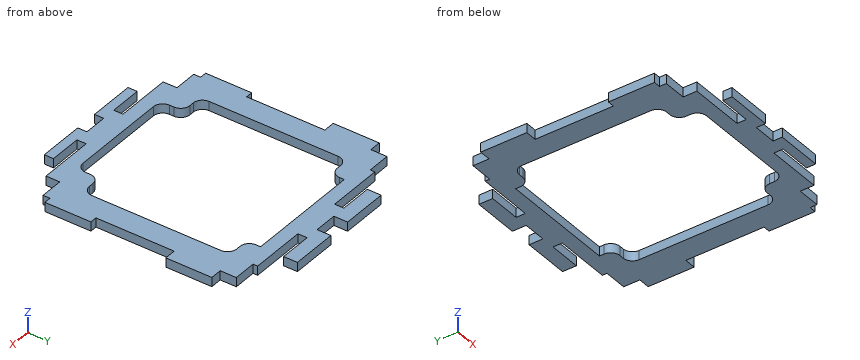
```python
from build123d import *

# Parameters (mm, degrees)
EXTRUDE_1_DEPTH = 2


with BuildPart() as part:
    # Model → 凸台-拉伸1 (new body)
    with BuildSketch(Plane.XY):
        Polygon((1277.912077, 487.080631391), (1277.912077, 483.580631391), (1275.412077, 483.580631391), (1275.412077, 473.580631391), (1277.912077, 473.580631391), (1277.912077, 456.580631391), (1276.412077, 456.580631391), (1276.412077, 446.580631391), (1277.912077, 446.580631391), (1277.912077, 445.080631391), (1282.912077, 445.080631391), (1282.912077, 442.080631391), (1294.912077, 442.080631391), (1294.912077, 440.080631391), (1287.912077, 440.080631391), (1287.912077, 438.080631391), (1297.912077, 438.080631391), (1297.912077, 440.080631391), (1302.912077, 440.080631391), (1302.912077, 438.080631391), (1312.912077, 438.080631391), (1312.912077, 440.080631391), (1305.912077, 440.080631391), (1305.912077, 442.080631391), (1317.912077, 442.080631391), (1317.912077, 445.080631391), (1322.912077, 445.080631391), (1322.912077, 446.580631391), (1324.412077, 446.580631391), (1324.412077, 456.580631391), (1322.912077, 456.580631391), (1322.912077, 473.580631391), (1325.412077, 473.580631391), (1325.412077, 483.580631391), (1322.912077, 483.580631391), (1322.912077, 487.080631391), (1317.912077, 487.080631391), (1317.912077, 488.080631391), (1305.912077, 488.080631391), (1305.912077, 490.080631391), (1312.912077, 490.080631391), (1312.912077, 493.080631391), (1302.912077, 493.080631391), (1302.912077, 490.080631391), (1297.912077, 490.080631391), (1297.912077, 493.080631391), (1287.912077, 493.080631391), (1287.912077, 490.080631391), (1294.912077, 490.080631391), (1294.912077, 488.080631391), (1282.912077, 488.080631391), (1282.912077, 487.080631391), align=None)
        with BuildLine():
            Line((1284.912077, 482.080631391), (1285.912077, 482.080631391))
            ThreePointArc((1285.912077, 482.080631391), (1287.326290562, 482.666417828), (1287.912077, 484.080631391))
            Line((1287.912077, 484.080631391), (1287.912077, 485.080631391))
            Line((1287.912077, 485.080631391), (1312.912077, 485.080631391))
            Line((1312.912077, 485.080631391), (1312.912077, 484.080631391))
            ThreePointArc((1312.912077, 484.080631391), (1313.497863438, 482.666417828), (1314.912077, 482.080631391))
            Line((1314.912077, 482.080631391), (1315.912077, 482.080631391))
            ThreePointArc((1315.912077, 482.080631391), (1317.326290562, 481.494844953), (1317.912077, 480.080631391))
            Line((1317.912077, 480.080631391), (1317.912077, 452.080631391))
            ThreePointArc((1317.912077, 452.080631391), (1317.326290562, 450.666417828), (1315.912077, 450.080631391))
            Line((1315.912077, 450.080631391), (1314.912077, 450.080631391))
            ThreePointArc((1314.912077, 450.080631391), (1313.497863438, 449.494844953), (1312.912077, 448.080631391))
            Line((1312.912077, 448.080631391), (1312.912077, 447.080631391))
            ThreePointArc((1312.912077, 447.080631391), (1312.326290562, 445.666417828), (1310.912077, 445.080631391))
            Line((1310.912077, 445.080631391), (1289.912077, 445.080631391))
            ThreePointArc((1289.912077, 445.080631391), (1288.497863438, 445.666417828), (1287.912077, 447.080631391))
            Line((1287.912077, 447.080631391), (1287.912077, 448.080631391))
            ThreePointArc((1287.912077, 448.080631391), (1287.326290562, 449.494844953), (1285.912077, 450.080631391))
            Line((1285.912077, 450.080631391), (1284.912077, 450.080631391))
            ThreePointArc((1284.912077, 450.080631391), (1283.497863438, 450.666417828), (1282.912077, 452.080631391))
            Line((1282.912077, 452.080631391), (1282.912077, 480.080631391))
            ThreePointArc((1282.912077, 480.080631391), (1283.497863438, 481.494844953), (1284.912077, 482.080631391))
        make_face(mode=Mode.SUBTRACT)
    extrude(amount=EXTRUDE_1_DEPTH)


solid = part.part
```
Design review of the part built by this model. Coordinates are the model's own, in mm. Round coordinates to 2 decimals unless told otherwise and drop trailing zeros. Write each loop counter-clockwise with the first axis right and the second up, starting at its lowest first coordinate (ties: lowest second). Pieces come first, ordered by that corner, then holes. Notation, with made-up numbers: (28.25, -3.75) -> (69.25, -3.75) arc R8 ccw to (69.25, 5.25) -> close; hole circle Ø3 at (-36, 79.25). An arc over 180 degrees is marked (long way). Answer in a Markdown table with one row per item.
Q1. Take a section at B-B, the plane x = 1309.5. State the section outline as (y, z) points, then the cut area to 3 significant figures.
The answers:
| item | result |
|---|---|
| outline | (438.08, 0) -> (440.08, 0) -> (440.08, 2) -> (438.08, 2) -> close; (442.08, 0) -> (445.08, 0) -> (445.08, 2) -> (442.08, 2) -> close; (485.08, 0) -> (488.08, 0) -> (488.08, 2) -> (485.08, 2) -> close; (490.08, 0) -> (493.08, 0) -> (493.08, 2) -> (490.08, 2) -> close |
| area | 22.0 mm² |
Q2. Take a section at C-C, the plane x = 1319. State the section outline as (y, z) points.
The answers:
| item | result |
|---|---|
| outline | (445.08, 0) -> (487.08, 0) -> (487.08, 2) -> (445.08, 2) -> close |
Q3. Take a section at A-A, the plane x = 1300. State the section outline as (y, z) points, then the cut area to 3 significant figures.
The answers:
| item | result |
|---|---|
| outline | (440.08, 0) -> (445.08, 0) -> (445.08, 2) -> (440.08, 2) -> close; (485.08, 0) -> (490.08, 0) -> (490.08, 2) -> (485.08, 2) -> close |
| area | 20.0 mm² |
Q4. Clearance check with flat-ended pins moving along their axes: pin 1 Ø1 at (x, z) = (1280, 1) entering from -Y; pin 2 Ø0.6 at (y, z) = (452.5, 1) entering from -X; pin 3 Ø1 at (y, z) = (467.5, 1) entering from -X. State where each tip first meets the part, or that it passes through.
The answers:
| item | result |
|---|---|
| pin 1 | y = 445.08 |
| pin 2 | x = 1276.41 |
| pin 3 | x = 1277.91 |
Q5. To check wall thickness, follow L1, parallel to Y at x = 1293, z = 1.4; L2, parallel to Y at x = 1295, z = 1.65; L3, parallel to Y at x = 1298, z = 0.4. State the ranges of each line that lie inside material, in increasing order. Write a range as [from, to].
The answers:
| item | result |
|---|---|
| L1 | [438.08, 440.08], [442.08, 445.08], [485.08, 488.08], [490.08, 493.08] |
| L2 | [438.08, 445.08], [485.08, 493.08] |
| L3 | [440.08, 445.08], [485.08, 490.08] |
